from build123d import *

# Parameters (mm, degrees)
SKETCH1_W                                    = 7
SKETCH1_H                                    = 4.7
BOSS_EXTRUDE1_DEPTH                          = 115
CUT_EXTRUDE1_DEPTH                           = 116
CBORE_FOR_SOCKET_HEAD_CAP_SCREW1_D           = 2.4
CBORE_FOR_SOCKET_HEAD_CAP_SCREW1_CBORE_D     = 4.2
CBORE_FOR_SOCKET_HEAD_CAP_SCREW1_CBORE_DEPTH = 2.3
LPATTERN1_COUNT                              = 8
LPATTERN1_PITCH                              = 15
CHAMFER1_SIZE                                = 0.3
CHAMFER2_SIZE                                = 0.3


with BuildPart() as part:
    # Sketch1 → Boss-Extrude1 (new body)
    with BuildSketch(Plane(origin=(-5, 0, 0), x_dir=(0, 0, -1), z_dir=(1, 0, 0))):
        with Locations((0, 2.35)):
            Rectangle(SKETCH1_W, SKETCH1_H)
    extrude(amount=BOSS_EXTRUDE1_DEPTH)

    # Sketch2 → Cut-Extrude1 (cut, through all)
    with BuildSketch(Plane(origin=(-5, 0, 0), x_dir=(0, 0, -1), z_dir=(1, 0, 0))):
        with BuildLine():
            Line((3.5, 4.034892917), (3.27, 3.902102355))
            ThreePointArc((3.27, 3.902102355), (3.075750359, 3.750022453), (2.931347317, 3.55))
            Line((2.931347317, 3.55), (2.2, 3.55))
            Line((2.2, 3.55), (2.2, 2.85))
            Line((2.2, 2.85), (2.931347317, 2.85))
            ThreePointArc((2.931347317, 2.85), (3.075750359, 2.649977547), (3.27, 2.497897645))
            Line((3.27, 2.497897645), (3.5, 2.365107083))
            Line((3.5, 2.365107083), (3.5, 4.034892917))
        make_face()
        with BuildLine():
            Line((-3.5, 4.034892917), (-3.5, 2.365107083))
            Line((-3.5, 2.365107083), (-3.27, 2.497897645))
            ThreePointArc((-3.27, 2.497897645), (-3.075750359, 2.649977547), (-2.931347317, 2.85))
            Line((-2.931347317, 2.85), (-2.2, 2.85))
            Line((-2.2, 2.85), (-2.2, 3.55))
            Line((-2.2, 3.55), (-2.931347317, 3.55))
            ThreePointArc((-2.931347317, 3.55), (-3.075750359, 3.750022453), (-3.27, 3.902102355))
            Line((-3.27, 3.902102355), (-3.5, 4.034892917))
        make_face()
    extrude(amount=CUT_EXTRUDE1_DEPTH, mode=Mode.SUBTRACT)

    # CBORE for Socket Head Cap Screw1 (through all)
    with Locations(Plane(origin=(0, 4.7, 0), x_dir=(1, 0, 0), z_dir=(0, 1, 0))):
        with Locations((0, 0)):
            cbore_for_socket_head_cap_screw1 = CounterBoreHole(CBORE_FOR_SOCKET_HEAD_CAP_SCREW1_D / 2, CBORE_FOR_SOCKET_HEAD_CAP_SCREW1_CBORE_D / 2, CBORE_FOR_SOCKET_HEAD_CAP_SCREW1_CBORE_DEPTH)

    # LPattern1: CBORE for Socket Head Cap Screw1 ×8
    with Locations(*[(i * LPATTERN1_PITCH, 0, 0) for i in range(1, LPATTERN1_COUNT)]):
        add(cbore_for_socket_head_cap_screw1, mode=Mode.SUBTRACT)

    # Chamfer1
    chamfer1_edges = [part.edges().sort_by_distance(p)[0] for p in [
        (52.5, 4.7, 3.5),
        (52.5, 4.7, -3.5),
    ]]
    chamfer(chamfer1_edges, length=CHAMFER1_SIZE)

    # Chamfer2
    chamfer2_edges = [part.edges().sort_by_distance(p)[0] for p in [
        (52.5, 0, -3.5),
        (52.5, 0, 3.5),
    ]]
    chamfer(chamfer2_edges, length=CHAMFER2_SIZE)


solid = part.part
Part model, mm, in its own coordinate system. A direction names the side the tool comes from. Coordinates: 2 decimals unless noted, no trailing zeros. Order: outer loops, then holes, each group sorted by start corner. A loop starts at its lowest first (then second) coordinate and runs counter-clockwise, first axis right, second up.
(1) Pin check, flat tip, straight feed: pin 1 Ø3 at (x, z) = (60, 0) entering from +Y. Stop position of the tip, or through.
Check sheet entries:
pin 1: stops at y = 2.4
(2) Pull direction Z, two halves, no side cores. Call faces 1 (the face through (105.95, 1.18, 0.73)), 2 (the face through (-5, 2, 0)), 3 (the face through (52, 1, -3.5)): pulls with the +Z half, pulls with the -Z half, needs draft (parallel to the pull), parting line crosses it, or undercut.
Check sheet entries:
face 1: undercut
face 2: needs draft
face 3: pulls with the -Z half
(3) Probe L1, parallel to Y at x = 76.5, z = 2.75; L2, parallel to Z at x = 75, y = 1.75; L3, parallel to Z at x = 105, y = 3.9. List the from-to ranges inside material, lowest first.
Check sheet entries:
L1: y = 0 to 2.85, 3.55 to 4.7
L2: z = -3.5 to -1.2, 1.2 to 3.5
L3: z = -3.27 to -2.1, 2.1 to 3.27
(4) Tool access for faces 4 (the face through (61.94, 3.57, 0.8)), 5 (the face through (28.89, 1.18, 0.46)): list every direction of +Z, -Z, +X, -X, +Y, -Y with a clear straight run to the whole face (end or side of a thin tool).
Check sheet entries:
face 4: +Y
face 5: +Y, -Y
(5) Slice it at B-B, the plane x = 6.5. Write the cut outline in (y, z).
Check sheet entries:
outline: (0, -3.2) - (0.3, -3.5) - (2.37, -3.5) - (2.5, -3.27) arc R0.88 cw to (2.85, -2.93) - (2.85, -2.2) - (3.55, -2.2) - (3.55, -2.93) arc R0.88 cw to (3.9, -3.27) - (4.03, -3.5) - (4.4, -3.5) - (4.7, -3.2) - (4.7, 3.2) - (4.4, 3.5) - (4.03, 3.5) - (3.9, 3.27) arc R0.88 cw to (3.55, 2.93) - (3.55, 2.2) - (2.85, 2.2) - (2.85, 2.93) arc R0.88 cw to (2.5, 3.27) - (2.37, 3.5) - (0.3, 3.5) - (0, 3.2) - close
